from build123d import *

# Parameters (mm, degrees)
SKETCH4_W           = 70
SKETCH4_H           = 120
BOSS_EXTRUDE2_DEPTH = 20


with BuildPart() as part:
    # Sketch4 → Boss-Extrude2 (new body)
    with BuildSketch(Plane(origin=(0, 0, 0), x_dir=(1, 0, 0), z_dir=(0, 1, 0))):
        Polygon((-100, 150), (100, 150), (100, 80), (190, 80), (190, -80), (100, -80), (100, -150), (-100, -150), (-100, -80), (-190, -80), (-190, 80), (-100, 80), align=None)
        with Locations((135, 0)):
            Rectangle(SKETCH4_W, SKETCH4_H, mode=Mode.SUBTRACT)
        Polygon((-80, 130), (-10, 130), (10, 130), (80, 130), (80, 60), (80, 40), (80, -40), (80, -60), (80, -130), (10, -130), (-10, -130), (-80, -130), (-80, -60), (-80, -40), (-80, 40), (-80, 60), align=None, mode=Mode.SUBTRACT)
        with Locations((-135, 0)):
            Rectangle(SKETCH4_W, SKETCH4_H, mode=Mode.SUBTRACT)
    extrude(amount=BOSS_EXTRUDE2_DEPTH)


solid = part.part
Source: CAD feature listing. Evaluate the final solid. Frame: model axes, mm. A direction names the side the tool comes from. Give positions to 0.01 mm unless a question says otherwise; leave off trailing zeros. Write each loop counter-clockwise with the first axis right and the second up, starting at its lowest first coordinate (ties: lowest second). Pieces come first, ordered by that corner, then holes. Notation, with made-up numbers: (87.25, -4) -> (128.25, -4) arc R10 cw to (128.25, 7) -> close; hole circle Ø3 at (-33.5, 32.25). An arc over 180 degrees is marked (long way). Return JSON: item names as keys, results as strings. Group by question number.
1. Mould query, pull axis Z, two halves, no side actions, for faces 5 (the face through (-100, 10, -115)), 6 (the face through (1, 10, 150)), 7 (the face through (-80, 10, 2)). Classes: +Z half, -Z half, draft (parallel to the pull), parting line (faces both ways), or undercut.
2. Material intervals for line 1 (X direction, y = 5.25, z = 14); line 2 (Z direction, x = -132.5, y = 5.5); line 3 (X direction, y = 12, z = 118.5), sorted ascending. Write a range as from..to.
3. Section B-B, the plane y = 3.25. Output: boundary loops of the cut face in (x, z).
4. Pin query (flat end, axial travel): pin 1 Ø2 at (y, z) = (2.5, 86) entering from -X; pin 2 Ø10 at (x, y) = (129, 8.5) entering from -Z. Return the tip coordinate at first contact, or that it passes through.
5. Section A-A, the plane z = -89. Output: boundary loops of the cut face in (x, y).
6. Section C-C, the plane x = 32. Output: boundary loops of the cut face in (y, z), then the cut area to 3 significant figures.
7. Section D-D, the plane z = 54. Output: boundary loops of the cut face in (x, y).
8. Access query for faces 1 (the face through (144, 10, -80)), 2 (the face through (1, 10, 130)), 3 (the face through (146, 10, 80)), 4 (the face through (-100, 10, 115)). Directions: +Z, -Z, +X, -X, +Y, -Y. A direction counts if a zero-diameter tool reaches every point of the face in a straight line with its end or side. Return the directions, or none.
Determined:
{
 "1": {"face 5": "draft", "face 6": "+Z half", "face 7": "undercut"},
 "2": {"line 1": "x = -190..-170, -100..-80, 80..100, 170..190", "line 2": "z = -80..-60, 60..80", "line 3": "x = -100..-80, 80..100"},
 "3": {"outline": "(-190, -80) -> (-100, -80) -> (-100, -150) -> (100, -150) -> (100, -80) -> (190, -80) -> (190, 80) -> (100, 80) -> (100, 150) -> (-100, 150) -> (-100, 80) -> (-190, 80) -> close; hole (-170, -60) -> (-100, -60) -> (-100, 60) -> (-170, 60) -> close; hole (-80, -130) -> (80, -130) -> (80, 130) -> (-80, 130) -> close; hole (100, -60) -> (170, -60) -> (170, 60) -> (100, 60) -> close"},
 "4": {"pin 1": "stops at x = -100", "pin 2": "stops at z = -80"},
 "5": {"outline": "(-100, 0) -> (-80, 0) -> (-80, 20) -> (-100, 20) -> close; (80, 0) -> (100, 0) -> (100, 20) -> (80, 20) -> close"},
 "6": {"outline": "(0, -150) -> (20, -150) -> (20, -130) -> (0, -130) -> close; (0, 130) -> (20, 130) -> (20, 150) -> (0, 150) -> close", "area": "800 mm2"},
 "7": {"outline": "(-190, 0) -> (-170, 0) -> (-170, 20) -> (-190, 20) -> close; (-100, 0) -> (-80, 0) -> (-80, 20) -> (-100, 20) -> close; (80, 0) -> (100, 0) -> (100, 20) -> (80, 20) -> close; (170, 0) -> (190, 0) -> (190, 20) -> (170, 20) -> close"},
 "8": {"face 1": "-Z, +X, +Y, -Y", "face 2": "+Y, -Y", "face 3": "+Z, +X, +Y, -Y", "face 4": "+Z, -X, +Y, -Y"}
}
